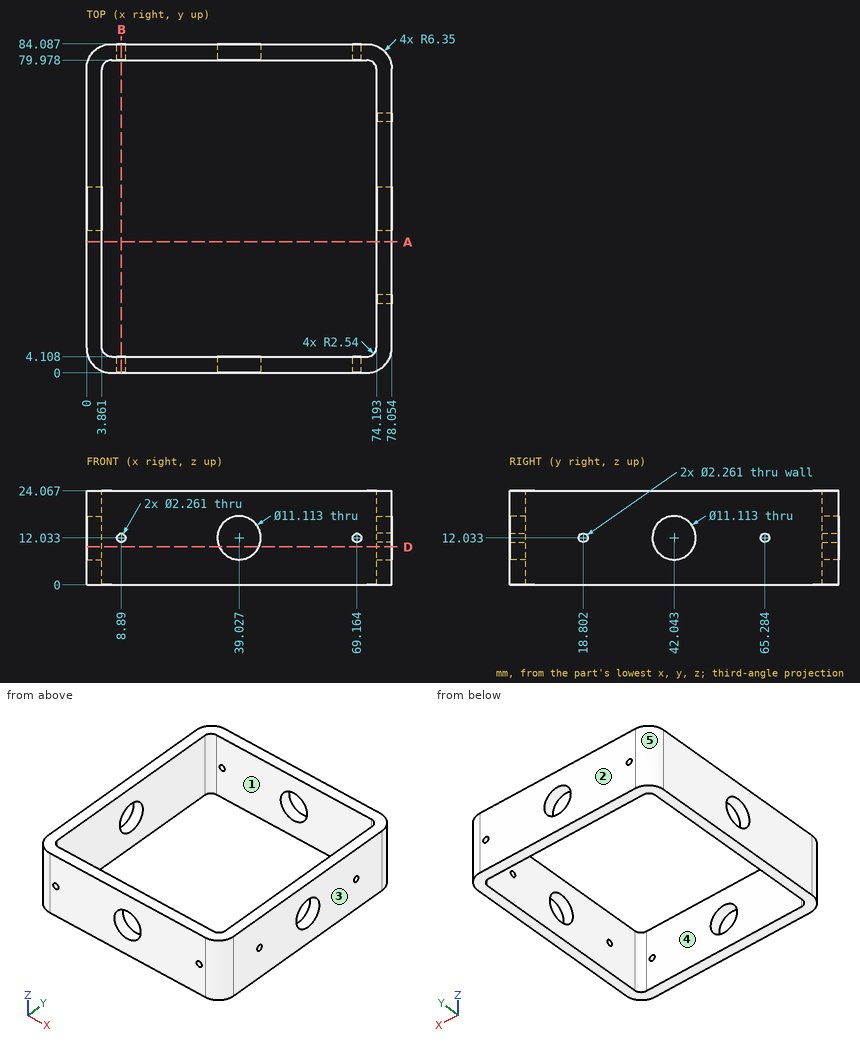
For this review, use the dimensioned drawing (mm, ordinates from the lowest corner) and the shaded views. A direction names the side the tool comes from. Give positions to 0.01 mm unless a question says otherwise; leave off trailing zeros. Write each loop counter-clockwise with the first axis right and the second up, starting at its lowest first coordinate (ties: lowest second). Pieces come first, ordered by that corner, then holes.
(1) For P1, Ø10, axis at y = 42.04, z = 12.03, coming from the -X side, flat-tipped, find the tip position at first contact; note if it passes through.
(2) Consider section A-A, the plane y = 33.5. Give the boundary of the cut face in (x, z) (1 decimal).
(3) To check wall thickness, follow L1, parallel to Z at x = 8.89, y = 1.8; L2, parallel to Y at x = 35, z = 22.75; L3, parallel to X at y = 50.5, z = 5.25 (1 decimal). State the ranges of each line that lie inside material, in increasing order.
(4) Consider section B-B, the plane x = 8.89. Give the boundary of the cut face in (y, z), and give its area (3 significant figures).
(5) Consider section D-D, the plane z = 9.75. Give the number of separate pieces and of enclosed holes in the cut face, and give its area (3 significant figures).
(6) The part is to be moulded in two halves that separate along Y. For the marked faces 1, 2 and 3, say which applies: released by +Y, released by -Y, zero draft, split by the parting line, or undercut.
(7) Tool access review of the marked faces 4 and 5: name each direction out of +Z, -Z, +X, -X, +Y, -Y from which nothing blocks a thin tool from reaching the whole face with its end or side.
Returned:
1. P1: passes through
2. outline: (0, 0) - (3.9, 0) - (3.9, 24.1) - (0, 24.1) - close; (74.2, 0) - (78.1, 0) - (78.1, 24.1) - (74.2, 24.1) - close
3. L1: z = 0 to 10.9, 13.16 to 24.07
3. L2: y = 0 to 4.11, 79.98 to 84.09
3. L3: x = 0 to 3.9, 74.2 to 78.1
4. outline: (0, 0) - (4.11, 0) - (4.11, 10.9) - (0, 10.9) - close; (0, 13.16) - (4.11, 13.16) - (4.11, 24.07) - (0, 24.07) - close; (79.98, 0) - (84.09, 0) - (84.09, 10.9) - (79.98, 10.9) - close; (79.98, 13.16) - (84.09, 13.16) - (84.09, 24.07) - (79.98, 24.07) - close
4. area: 179 mm2
5. separate pieces: 4
5. enclosed holes: 0
5. area: 1,040 mm2
6. face 1: undercut
6. face 2: released by +Y
6. face 3: zero draft
7. face 4: +Z, -Z
7. face 5: +Z, -Z, -X, +Y
